from build123d import *

# Parameters (mm, degrees)
SKETCH1_R           = 9.5
BOSS_EXTRUDE1_DEPTH = 10
CHAMFER1_SIZE       = 2
SKETCH2_R           = 13
BOSS_EXTRUDE2_DEPTH = 3
BOSS_EXTRUDE3_DEPTH = 3.5
BOSS_EXTRUDE3_TAPER = 8
FILLET1_R           = 1
SKETCH3_W           = 2.290416552
SKETCH3_H           = 4.294163917
CUT_EXTRUDE1_DEPTH  = 1


with BuildPart() as part:
    # Sketch1 → Boss-Extrude1 (new body)
    with BuildSketch(Plane.XY):
        Circle(SKETCH1_R)
    extrude(amount=BOSS_EXTRUDE1_DEPTH)

    # Chamfer1
    chamfer1_edges = [part.edges().sort_by_distance(p)[0] for p in [
        (-9.5, 0, 0),
    ]]
    chamfer(chamfer1_edges, length=CHAMFER1_SIZE)

    # Sketch2 → Boss-Extrude2 (add)
    with BuildSketch(Plane.XY.offset(10)):
        Circle(SKETCH2_R)
    extrude(amount=BOSS_EXTRUDE2_DEPTH)

    # Sketch4 → Boss-Extrude3 (add)
    with BuildSketch(Plane.XY.offset(13)):
        with BuildLine():
            ThreePointArc((3, 10.583005244), (0, 11), (-3, 10.583005244))
            Line((-3, 10.583005244), (-3, 4))
            ThreePointArc((-3, 4), (0, 5), (3, 4))
            Line((3, 4), (3, 10.583005244))
        make_face()
        with BuildLine():
            ThreePointArc((3, -4), (0, -5), (-3, -4))
            Line((-3, -4), (-3, -10.583005244))
            ThreePointArc((-3, -10.583005244), (0, -11), (3, -10.583005244))
            Line((3, -10.583005244), (3, -4))
        make_face()
    extrude(amount=BOSS_EXTRUDE3_DEPTH, taper=BOSS_EXTRUDE3_TAPER)

    # Fillet1
    fillet1_edges = [part.edges().sort_by_distance(p)[0] for p in [
        (-13, 0, 10),
        (-13, 0, 13),
    ]]
    fillet(fillet1_edges, radius=FILLET1_R)

    # Sketch3 → Cut-Extrude1 (cut)
    with BuildSketch(Plane.XY.offset(13)):
        Polygon((-1.625120105, -2.013905208), (-1.625120105, -1.413905208), (-0.367640206, -1.413905208), (-0.367640206, 2.880258709), (-1.625120105, 2.880258709), (-1.625120105, 3.480258709), (1.874879895, 3.480258709), (1.874879895, 2.880258709), (0.367640206, 2.880258709), (0.367640206, -1.413905208), (1.874879895, -1.413905208), (1.874879895, -2.013905208), align=None)
        Polygon((5.359789492, 3.480258709), (5.359789492, -1.419741291), (5.359789492, -2.019741291), (8.274879895, -2.019741291), (8.274879895, -1.419741291), (5.974879895, -1.419741291), (5.974879895, 3.480258709), align=None)
        Polygon((-8.615536657, 3.480258709), (-8.615536657, -2.013905208), (-5.125120105, -2.013905208), (-5.125120105, 2.880258709), (-5.125120105, 3.480258709), align=None)
        with Locations((-6.870328381, 0.73317675)):
            Rectangle(SKETCH3_W, SKETCH3_H, mode=Mode.SUBTRACT)
    extrude(amount=-CUT_EXTRUDE1_DEPTH, mode=Mode.SUBTRACT)


solid = part.part
For this review, take the finished solid that the model builds, in its own axes (mm). A direction names the side the tool comes from. Coordinates: 2 decimals unless noted, no trailing zeros. Order: outer loops, then holes, each group sorted by start corner. A loop starts at its lowest first (then second) coordinate and runs counter-clockwise, first axis right, second up. Notation, with made-up numbers: (79, 10) -> (95, 10) arc R8 cw to (95, 20) -> close; hole circle Ø11 at (63, 39). An arc over 180 degrees is marked (long way). Return JSON: item names as keys, results as strings.
1. For pin 1 Ø0.8 at (y, z) = (0.5, 12.5) entering from +X; pin 2 Ø6 at (x, y) = (-9, 7.5) entering from +Z; pin 3 Ø0.8 at (x, z) = (-1, 12.5) entering from +Y, all flat-tipped, find the tip position at first contact; note any pin that passes through.
Answer block:
{"pin 1": "x = 12.99", "pin 2": "z = 13", "pin 3": "y = 12.96"}
2. We need section B-B on x = 0. Write out the cut boundary in (y, z).
Answer block:
{"outline": "(-13, 11) arc R1 ccw to (-12, 10) -> (-9.5, 10) -> (-9.5, 2) -> (-7.5, 0) -> (7.5, 0) -> (9.5, 2) -> (9.5, 10) -> (12, 10) arc R1 ccw to (13, 11) -> (13, 12) arc R1 ccw to (12, 13) -> (11, 13) -> (10.51, 16.5) -> (5.49, 16.5) -> (5, 13) -> (3.48, 13) -> (3.48, 12) -> (-2.01, 12) -> (-2.01, 13) -> (-5, 13) -> (-5.49, 16.5) -> (-10.51, 16.5) -> (-11, 13) -> (-12, 13) arc R1 ccw to (-13, 12) -> close"}
3. For line 1 (Z direction, x = -7, y = -1); line 2 (X direction, y = 0.25, z = 9.5); line 3 (Y direction, x = 10, z = 10.75), list the stretches that pass through material, from the lowest coordinate up. Write a range as from..to.
Answer block:
{"line 1": "0..13", "line 2": "-9.5..9.5", "line 3": "-8.26..8.26"}
4. We need section D-D on z = 1.5. Write out the cut boundary in (x, y), and give its area (3 significant figures).
Answer block:
{"outline": "circle Ø18 at (0, 0)", "area": "254 mm²"}
5. We need section A-A on z = 14.25. Write out the cut boundary in (x, y), and give its area (3 significant figures).
Answer block:
{"outline": "(-2.82, -10.45) arc R10.82 ccw to (2.82, -10.45) -> (2.82, -4.34) arc R5.18 cw to (-2.82, -4.34) -> close; (-2.82, 4.34) arc R5.18 cw to (2.82, 4.34) -> (2.82, 10.45) arc R10.82 ccw to (-2.82, 10.45) -> close", "area": "65.5 mm²"}
6. The part is to be moulded in two halves that separate along Y. For faces 1 (the conical face through (-0.04, -10.75, 14.77)), 2 (the flat face through (2.757, -7.245, 14.726)), 3 (the conical face through (-0.05, 5.25, 14.77)), 4 (the flat face through (1.1, -1.414, 12.5)), say which applies: +Y half, -Y half, draft (parallel to the pull), parting line (faces both ways), or undercut.
Answer block:
{"face 1": "-Y half", "face 2": "draft", "face 3": "undercut", "face 4": "undercut"}
7. Machinability: for faces 5 (the flat face through (9, 4, 10)), 6 (the flat face through (2.757, 7.338, 14.726)), 7 (the flat face through (7.1, -1.42, 12.5)), which of the approach directions +Z, -Z, +X, -X, +Y, -Y give a long, thin tool a straight path to every point of the face, cutting with its end or side? Answer none if there is none.
Answer block:
{"face 5": "-Z", "face 6": "+Z, +X, +Y, -Y", "face 7": "+Z"}
